```python
from build123d import *

# Parameters (mm, degrees)
SKETCH1_W           = 71
SKETCH1_H           = 20
BOSS_EXTRUDE1_DEPTH = 5
SKETCH2_R           = 2.95
CUT_EXTRUDE1_DEPTH  = 5
CHAMFER1_SIZE       = 1.6
SKETCH3_W           = 36
SKETCH3_H           = 13
BOSS_EXTRUDE2_DEPTH = 14.3
BOSS_EXTRUDE3_DEPTH = 13
CHAMFER2_START      = -20.499775095
CHAMFER2_OUTLINE_W  = 14.439182802
CHAMFER2_OUTLINE_H  = 13
CHAMFER2_DEPTH      = 2.499775095
CHAMFER3_START      = 18
CHAMFER3_OUTLINE_W  = 14.439182802
CHAMFER3_OUTLINE_H  = 13
CHAMFER3_DEPTH      = 2.499775095
SKETCH6_R           = 2.2
CUT_EXTRUDE2_DEPTH  = 12
FILLET2_R           = 3
FILLET3_R           = 5


with BuildPart() as part:
    # Sketch1 → Boss-Extrude1 (new body)
    with BuildSketch(Plane(origin=(0, 0, 0), x_dir=(1, 0, 0), z_dir=(0, 1, 0))):
        Rectangle(SKETCH1_W, SKETCH1_H)
    extrude(amount=BOSS_EXTRUDE1_DEPTH)

    # Sketch2 → Cut-Extrude1 (cut)
    with BuildSketch(Plane(origin=(0, 5, 0), x_dir=(1, 0, 0), z_dir=(0, 1, 0))):
        with Locations(Location((28, 0, 0), (0, 0, 270))):
            Circle(SKETCH2_R)
        with Locations(Location((-28, 0, 0), (0, 0, 270))):
            Circle(SKETCH2_R)
    extrude(amount=-CUT_EXTRUDE1_DEPTH, mode=Mode.SUBTRACT)

    # Chamfer1
    chamfer1_edges = [part.edges().sort_by_distance(p)[0] for p in [
        (28, 5, -2.95),
        (-28, 5, -2.95),
    ]]
    chamfer(chamfer1_edges, length=CHAMFER1_SIZE)

    # Sketch3 → Boss-Extrude2 (add)
    with BuildSketch(Plane(origin=(0, 5, 0), x_dir=(1, 0, 0), z_dir=(0, 1, 0))):
        with Locations((0, 3.5)):
            Rectangle(SKETCH3_W, SKETCH3_H)
    extrude(amount=BOSS_EXTRUDE2_DEPTH)

    # Sketch5 → Boss-Extrude3 (add)
    with BuildSketch(Plane(origin=(0, 0, -10), x_dir=(-1, 0, 0), z_dir=(0, 0, -1))):
        with BuildLine():
            Line((-18, 19.3), (18, 19.3))
            ThreePointArc((18, 19.3), (0, 37.3), (-18, 19.3))
        make_face()
    extrude(amount=-BOSS_EXTRUDE3_DEPTH)

    # Chamfer2: read off the stored shape, not the designer's step
    # Chamfer2 outline → Chamfer2 (add)
    with BuildSketch(Plane(origin=(0, 0, 0), x_dir=(0.13851199388326604, 0.9903607562653531, 0), z_dir=(0.9903607562653531, -0.13851199388326602, 0)).offset(CHAMFER2_START)):
        with Locations((9.401155305, -3.5)):
            Rectangle(CHAMFER2_OUTLINE_W, CHAMFER2_OUTLINE_H)
    extrude(amount=CHAMFER2_DEPTH)

    # Chamfer3: read off the stored shape, not the designer's step
    # Chamfer3 outline → Chamfer3 (add)
    with BuildSketch(Plane(origin=(0, 0, 0), x_dir=(-0.13851199388326604, 0.9903607562653531, 0), z_dir=(0.9903607562653531, 0.13851199388326602, 0)).offset(CHAMFER3_START)):
        with Locations((9.401155305, -3.5)):
            Rectangle(CHAMFER3_OUTLINE_W, CHAMFER3_OUTLINE_H)
    extrude(amount=CHAMFER3_DEPTH)

    # Sketch6 → Cut-Extrude2 (cut)
    with BuildSketch(Plane.XY.offset(3)):
        with Locations((0, 19.3)):
            Circle(SKETCH6_R)
    extrude(amount=-CUT_EXTRUDE2_DEPTH, mode=Mode.SUBTRACT)

    # Fillet2
    fillet2_edges = [part.edges().sort_by_distance(p)[0] for p in [
        (-20, 5, -3.5),
        (20, 5, -3.5),
    ]]
    fillet(fillet2_edges, radius=FILLET2_R)

    # Fillet3
    fillet3_edges = [part.edges().sort_by_distance(p)[0] for p in [
        (-1, 5, 3),
    ]]
    fillet(fillet3_edges, radius=FILLET3_R)


solid = part.part
```
Check sheet for the modelled part. Datum: model origin and axes. Units: mm. A direction names the side the tool comes from. Round coordinates to 2 decimals unless told otherwise and drop trailing zeros. Order: outer loops, then holes, each group sorted by start corner. A loop starts at its lowest first (then second) coordinate and runs counter-clockwise, first axis right, second up. Notation, with made-up numbers: (-25, 46.25) -> (18, 46.25) arc R27 ccw to (18, 78.25) -> close; hole circle Ø8 at (-5, 29.25). An arc over 180 degrees is marked (long way). Use CSV: the item, a comma, the result in double quotes.
(1) Material ranges on line 1 along X through (y, z) = (2, 0); line 2 along Y through (x, z) = (0, -4); line 3 along X through (y, z) = (3, 1.75), recorded low to high. Write a range as from..to.
Worked out:
line 1,"-35.5..-30.95, -25.05..25.05, 30.95..35.5"
line 2,"0..17.1, 21.5..37.3"
line 3,"-35.5..-30.37, -25.63..25.63, 30.37..35.5"
(2) Cross-section at B-B (x = 0). Record the boundary of the cut face in (y, z), and give its area (3 significant figures).
Worked out:
outline,"(0, -10) -> (37.3, -10) -> (37.3, 3) -> (21.5, 3) -> (21.5, -9) -> (17.1, -9) -> (17.1, 3) -> (10, 3) arc R5 cw to (5, 8) -> (5, 10) -> (0, 10) -> close"
area,"472 mm²"
(3) Tool access check on faces 4 (the face through (0, 15, -10)), 5 (the face through (0, 24, 3)), 6 (the face through (1.02, 17.35, -2.92)). Record the directions out of +Z, -Z, +X, -X, +Y, -Y that give a thin tool (end or side, any length) a straight path to the whole face; none if there is none.
Worked out:
face 4,"-Z, +X, -X, +Y, -Y"
face 5,"+Z, +X, -X, +Y"
face 6,"+Z"
(4) Depth check by flat-ended pin: pin 1 (12 mm diameter, centred on x = -28, y = 27.5, fed in from +Z); pin 2 (5 mm diameter, centred on y = 10.5, z = -5, fed in from +X); pin 3 (7 mm diameter, centred on x = -28, z = 0, fed in from +Y); pin 4 (5 mm diameter, centred on x = -0.5, y = 18.5, fed in from +Z). Enter the tip coordinate at first touch or a pass-through.
Worked out:
pin 1,"through"
pin 2,"x = 19.58"
pin 3,"y = 3.95"
pin 4,"z = 3"
(5) Cross-section at A-A (x = -28). Record the boundary of the cut face in (y, z), and give its area (3 significant figures).
Worked out:
outline,"(0, -10) -> (5, -10) -> (5, -4.55) -> (3.4, -2.95) -> (0, -2.95) -> close; (0, 2.95) -> (3.4, 2.95) -> (5, 4.55) -> (5, 10) -> (0, 10) -> close"
area,"67.9 mm²"
(6) Draft check along X on faces 1 (the face through (-0.396, 37.296, -3.591)), 2 (the face through (0, 19, -9)), 3 (the face through (0, 5, 9)). Enter one of: pulls with the +X half, pulls with the -X half, needs draft (parallel to the pull), parting line crosses it, or undercut.
Worked out:
face 1,"parting line crosses it"
face 2,"undercut"
face 3,"needs draft"
(7) Cross-section at D-D (z = -1.5). Count the separate pieces of the cut face and the enclosed holes in it, and give its area (3 significant figures).
Worked out:
separate pieces,"3"
enclosed holes,"1"
area,"1,340 mm²"
(8) Cross-section at C-C (y = 20). Record the boundary of the cut face in (x, z), and give its area (3 significant figures).
Worked out:
outline,"(-17.99, -10) -> (17.99, -10) -> (17.99, 3) -> (2.09, 3) -> (2.09, -9) -> (-2.09, -9) -> (-2.09, 3) -> (-17.99, 3) -> close"
area,"418 mm²"
